Check sheet for the modelled part. Datum: model origin and axes. Units: mm. Face numbers are marked on the shaded views. Give positions to 0.01 mm unless a question says otherwise; leave off trailing zeros. Loops run counter-clockwise (first coordinate to the right, second up) from the corner with the lowest first, then second, coordinate; pieces in that order, holes last. Notation, with made-up numbers: (21.5, 67) - (49.5, 67) arc R15 cw to (49.5, 71) - close; hole circle Ø10 at (28.5, 78.5). An arc over 180 degrees is marked (long way). Answer in a Markdown table with one row per item. Add a question column.
(1) Go/stop test with flat-tipped pins: P1, Ø1.5, axis at x = 15.5, y = 783, coming from the +Z side; P2, Ø10, axis at x = -23.5, z = 29, coming from the +Y side; P3, Ø10, axis at x = -29.5, y = 152.5, coming from the +Z side. Record where each tip stops, or that it passes through.
(2) Thickness scan on L1, parallel to Y at x = 0, z = -7; L2, parallel to Z at x = -3, y = 512.5; L3, parallel to Z at x = -0.5, y = 122. Record the ranges inside material, lowest first.
(3) Sectioned sample at D-D on y = 248. Enter the section's corners in (x, z), then the cut area to 3 significant figures.
(4) Draft check along Y on the marked faces 1, 2 and 3. Enter one of: released by +Y, released by -Y, zero draft, split by the parting line, or undercut.
(5) Sectioned sample at A-A on x = 0. Enter the section's corners in (y, z), then the cut area to 3 significant figures.
(6) Sectioned sample at B-B on y = 1015. Enter the section's corners in (x, z).
(7) Sectioned sample at C-C on z = 0. Enter the section's corners in (x, y), then the cut area to 3 significant figures.
Solid Edge part; units mm, degrees
sketch "Sketch1" plane through (0, 0, 0) normal (0, -1, 0) x (1, 0, 0)
  circle A0 centre (0, 0) radius 30
extrude "Protrusion1" add sketch "Sketch1" against normal blind 1015
sketch "Sketch2" plane through (0, 0, 0) normal (0, 0, 1) x (1, 0, 0)
  circle A0 centre (0, 1015) radius 40
extrude "ExtrudedProtrusion_4" add sketch "Sketch2" along normal mid plane 80
sketch "Sketch3" plane through (0, 528, 40) normal (0, 0, 1) x (1, 0, 0)
  circle A0 centre (0, 487) radius 30
extrude "Cutout1" cut sketch "Sketch3" against normal through all
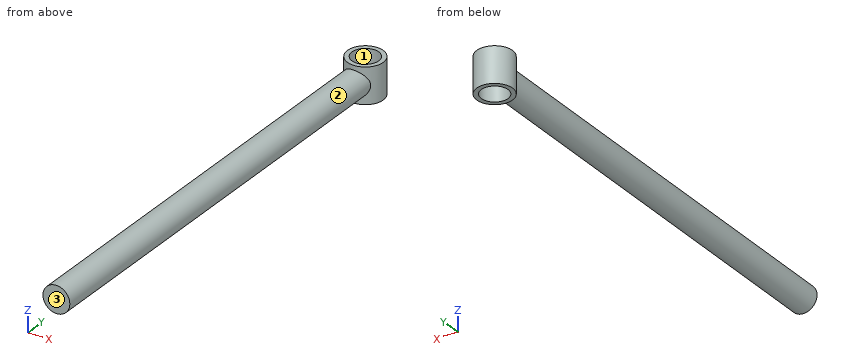
Reply:
| question | item | result |
|---|---|---|
| 1 | P1 | z = 26.12 |
| 1 | P2 | y = 1050.46 |
| 1 | P3 | z = 17.31 |
| 2 | L1 | 0 to 985, 1045 to 1055 |
| 2 | L2 | -29.85 to 29.85 |
| 2 | L3 | -30 to 30 |
| 3 | outline | circle Ø60 at (0, 0) |
| 3 | area | 2,830 mm^2 |
| 4 | face 1 | undercut |
| 4 | face 2 | zero draft |
| 4 | face 3 | released by -Y |
| 5 | outline | (0, -30) - (975, -30) - (975, -40) - (985, -40) - (985, 40) - (975, 40) - (975, 30) - (0, 30) - close; (1045, -40) - (1055, -40) - (1055, 40) - (1045, 40) - close |
| 5 | area | 60,100 mm^2 |
| 6 | outline | (-40, -40) - (-30, -40) - (-30, 40) - (-40, 40) - close; (30, -40) - (40, -40) - (40, 40) - (30, 40) - close |
| 7 | outline | (-30, 0) - (30, 0) - (30, 988.54) arc R40 ccw (long way) to (-30, 988.54) - close; hole circle Ø60 at (0, 1015) |
| 7 | area | 60,900 mm^2 |
